from build123d import *

# Parameters (mm, degrees)
BOSS_EXTRUDE2_DEPTH      = 4
BOSS_EXTRUDE3_DEPTH      = 25.13
SKETCH7_W                = 8
SKETCH7_H                = 3
BOSS_EXTRUDE4_DEPTH      = 25.13
SKETCH32_W               = 40.2
SKETCH32_H               = 6
BOSS_EXTRUDE6_DEPTH      = 20.93
SKETCH70_R               = 1.75
CUT_EXTRUDE23_DEPTH      = 5
SKETCH71_R               = 1.75
CUT_EXTRUDE24_DEPTH      = 6
CUT_EXTRUDE26_DEPTH      = 10
CUT_EXTRUDE26_DEPTH_BACK = 25
SKETCH86_R               = 1.25
SKETCH88_W               = 40.2
SKETCH88_H               = 4
BOSS_EXTRUDE26_DEPTH     = 6
CUT_EXTRUDE28_DEPTH      = 4
CUT_EXTRUDE28_DEPTH_BACK = 30
SKETCH89_R               = 1.25


# Read off the part's stored shape, not the designer's step: Boss-Extrude3
with BuildPart() as part:
    # Sketch5 → Boss-Extrude2 (new body)
    with BuildSketch(Plane.XY):
        Polygon((-138.644230049, -51.409116495), (-138.644230049, -41.159116495), (-146.644230049, -41.159116495), (-146.644230049, -38.159116495), (-138.644230049, -38.159116495), (-138.644230049, -14.059116495), (-98.444230049, -14.059116495), (-98.444230049, -38.159116495), (-90.444230049, -38.159116495), (-90.444230049, -41.159116495), (-98.444230049, -41.159116495), (-98.444230049, -51.409116495), align=None)
    extrude(amount=BOSS_EXTRUDE2_DEPTH)

    # Boss-Extrude3 outline → Boss-Extrude3 (add)
    with BuildSketch(Plane(origin=(0, 0, 0), x_dir=(-1, 0, 0), z_dir=(0, 0, -1))):
        Polygon((138.644230049, -38.159116495), (138.644230049, -41.159116495), (146.644230049, -41.159116495), (146.644230049, -38.165572531), align=None)
    extrude(amount=BOSS_EXTRUDE3_DEPTH)

    # Sketch7 → Boss-Extrude4 (add)
    with BuildSketch(Plane(origin=(0, 0, 0), x_dir=(-1, 0, 0), z_dir=(0, 0, -1))):
        with Locations((94.444230049, -39.659116495)):
            Rectangle(SKETCH7_W, SKETCH7_H)
    extrude(amount=BOSS_EXTRUDE4_DEPTH)

    # Sketch70 → Cut-Extrude23 (cut)
    with BuildSketch(Plane(origin=(0, -38.159116495, 0), x_dir=(1, 0, 0), z_dir=(0, 1, 0))):
        with Locations(Location((-93.644230062, 5.405, 0), (0, 0, 180))):
            Circle(SKETCH70_R)
        with Locations(Location((-93.644230062, 15.755, 0), (0, 0, 180))):
            Circle(SKETCH70_R)
    extrude(amount=-CUT_EXTRUDE23_DEPTH, mode=Mode.SUBTRACT)

    # Sketch71 → Cut-Extrude24 (cut)
    with BuildSketch(Plane(origin=(0, -41.159116495, 0), x_dir=(-1, 0, 0), z_dir=(0, -1, 0))):
        with Locations(Location((143.444230049, 15.755, 0), (0, 0, 90))):
            Circle(SKETCH71_R)
        with Locations(Location((143.444230049, 5.405, 0), (0, 0, 90))):
            Circle(SKETCH71_R)
    extrude(amount=-CUT_EXTRUDE24_DEPTH, mode=Mode.SUBTRACT)



with BuildPart() as body_2:
    # Sketch32 → Boss-Extrude6 (new body)
    with BuildSketch(Plane(origin=(0, 0, 0), x_dir=(-1, 0, 0), z_dir=(0, 0, -1))):
        with Locations((118.544230049, -11.059116495)):
            Rectangle(SKETCH32_W, SKETCH32_H)
    extrude(amount=BOSS_EXTRUDE6_DEPTH)

    # Sketch86 → Cut-Extrude26 (cut, two sides: drawn at the far end of the back side and taken through both)
    with BuildSketch(Plane(origin=(0, 0, -20.93), x_dir=(-1, 0, 0), z_dir=(0, 0, -1)).offset(-CUT_EXTRUDE26_DEPTH_BACK)):
        with Locations(Location((122.644230049, -11.0591165, 0), (0, 0, 180))):
            Circle(SKETCH86_R)
        with Locations(Location((114.644230049, -11.0591165, 0), (0, 0, 180))):
            Circle(SKETCH86_R)
        with Locations(Location((106.644230049, -11.0591165, 0), (0, 0, 180))):
            Circle(SKETCH86_R)
    extrude(amount=CUT_EXTRUDE26_DEPTH + CUT_EXTRUDE26_DEPTH_BACK, mode=Mode.SUBTRACT)


with BuildPart() as part_1:
    add(part.part)

    add(body_2.part)  # Boss-Extrude26 merges body 2
    # Sketch88 → Boss-Extrude26 (add)
    with BuildSketch(Plane(origin=(0, -14.059116495, 0), x_dir=(1, 0, 0), z_dir=(0, 1, 0))):
        with Locations((-118.544230049, -2)):
            Rectangle(SKETCH88_W, SKETCH88_H)
    extrude(amount=BOSS_EXTRUDE26_DEPTH)

    # Sketch89 → Cut-Extrude28 (cut, two sides: drawn at the far end of the back side and taken through both)
    with BuildSketch(Plane.XY.offset(4).offset(-CUT_EXTRUDE28_DEPTH_BACK)):
        with Locations(Location((-122.644230049, -11.059116495, 0), (0, 0, 359.999999768))):
            Circle(SKETCH89_R)
        with Locations(Location((-114.644230049, -11.059116495, 0), (0, 0, 359.999999768))):
            Circle(SKETCH89_R)
        with Locations((-130.636250743, -11.059116495)):
            Circle(SKETCH89_R)
        with Locations(Location((-106.644230049, -11.059116495, 0), (0, 0, 359.999999768))):
            Circle(SKETCH89_R)
    extrude(amount=CUT_EXTRUDE28_DEPTH + CUT_EXTRUDE28_DEPTH_BACK, mode=Mode.SUBTRACT)


solid = part_1.part
For this review, take the finished solid that the model builds, in its own axes (mm). A direction names the side the tool comes from. Coordinates: 2 decimals unless noted, no trailing zeros. Order: outer loops, then holes, each group sorted by start corner. A loop starts at its lowest first (then second) coordinate and runs counter-clockwise, first axis right, second up. Notation, with made-up numbers: (44.5, 34.5) - (69.5, 34.5) arc R14 ccw to (69.5, 48.5) - close; hole circle Ø4 at (-30.75, 21). An arc over 180 degrees is marked (long way). Use one line per item in the form item = value.
Q1. For P1, Ø10, axis at x = -139, y = -36.5, coming from the -Z side; P2, Ø3, axis at x = -143.44, z = -15.76, coming from the -Y side; P3, Ø3, axis at y = -44.5, z = 1, coming from the -X side; P4, Ø2, axis at y = -46.5, z = 1.5, coming from the +X side, all flat-tipped, find the tip position at first contact; note any pin that passes through.
Checked values:
P1 = -25.13
P2 = through
P3 = -138.64
P4 = -98.44
Q2. Consider section B-B (z = -16.5). Give the number of separate pieces and of enclosed holes in the cut face, then the cut area to 3 significant figures.
Checked values:
separate_pieces = 5
enclosed_holes = 4
area = 251 mm2
Q3. Consider section C-C (z = -21.75). Give the boundary of the cut face in (x, y), then the cut area to 3 significant figures.
Checked values:
outline = (-146.64, -41.16) - (-138.64, -41.16) - (-138.64, -38.16) - (-146.64, -38.17) - close; (-98.44, -41.16) - (-90.44, -41.16) - (-90.44, -38.16) - (-98.44, -38.16) - close
area = 48.0 mm2
Q4. For probe 1 along Y at (x, z) = (-106.5, -18.75); probe 2 along X at (y, z) = (-12, 1); probe 3 along Z at (x, y) = (-125, -42.5), list the stretches that pass through material, from the lowest coordinate up. Write a range as from..to.
Checked values:
probe_1 = -14.06..-12.3, -9.82..-8.06
probe_2 = -138.64..-131.46, -129.81..-123.47, -121.82..-115.47, -113.82..-107.47, -105.82..-98.44
probe_3 = 0..4
Q5. Consider section D-D (x = -107). Give the boundary of the cut face in (y, z), then the cut area to 3 significant figures.
Checked values:
outline = (-51.41, 0) - (-14.06, 0) - (-14.06, -20.93) - (-12.26, -20.93) - (-12.26, 4) - (-51.41, 4) - close; (-9.86, -20.93) - (-8.06, -20.93) - (-8.06, 4) - (-9.86, 4) - close
area = 239 mm2
Q6. Consider section A-A (z = -8.5). Give the boundary of the cut face in (x, y).
Checked values:
outline = (-146.64, -41.16) - (-138.64, -41.16) - (-138.64, -38.16) - (-146.64, -38.17) - close; (-138.64, -14.06) - (-98.44, -14.06) - (-98.44, -8.06) - (-138.64, -8.06) - close; (-98.44, -41.16) - (-90.44, -41.16) - (-90.44, -38.16) - (-98.44, -38.16) - close; hole circle Ø2.5 at (-130.64, -11.06); hole circle Ø2.5 at (-122.64, -11.06); hole circle Ø2.5 at (-114.64, -11.06); hole circle Ø2.5 at (-106.64, -11.06)
Q7. For faces 1 (the flat face through (-118, -14.059, -10)), 2 (the flat face through (-94, -41.159, -10)), 3 (the flat face through (-138.644, -13, -3)), 4 (the flat face through (-138.644, -40, -12)), list the 3-axis set-ups (+Z, -Z, +X, -X, +Y, -Y) from which the entire face can be reached by the end or side of a thin tool; tool diameter is ignored.
Checked values:
face_1 = -Z, +X, -X, -Y
face_2 = +Z, -Z, +X, -Y
face_3 = +Z, -Z, -X, +Y
face_4 = -Z, -Y
Q8. Draft analysis for pull direction X (two halves, no side actions). For faces 5 (the cylindrical face through (-95.313, -39.638, -15.229)), 6 (the flat face through (-94, -38.159, -10)), 7 (the flat face through (-146.644, -40, -10)), 8 (the cylindrical face through (-145, -39.68, -6.21)), state which applies: +X half, -X half, draft (parallel to the pull), parting line (faces both ways), or undercut.
Checked values:
face_5 = undercut
face_6 = draft
face_7 = -X half
face_8 = undercut
